```python
from build123d import *

# Parameters (mm, degrees)
SKETCH1_W           = 86.36
SKETCH1_H           = 86.36
BOSS_EXTRUDE1_DEPTH = 43.18
SKETCH2_W           = 81.28
SKETCH2_H           = 81.28
CUT_EXTRUDE2_DEPTH  = 35.56
SKETCH6_W           = 81.28
SKETCH6_H           = 81.28
SKETCH6_R           = 1.016
BOSS_EXTRUDE2_DEPTH = 30.48
SKETCH9_R           = 6.35
CUT_EXTRUDE3_DEPTH  = 5.08
CUT_EXTRUDE4_REACH  = 107.769
SKETCH10_R          = 1.905


with BuildPart() as part:
    # Sketch1 → Boss-Extrude1 (new body)
    with BuildSketch(Plane(origin=(0, 0, 0), x_dir=(1, 0, 0), z_dir=(0, 1, 0))):
        Rectangle(SKETCH1_W, SKETCH1_H)
    extrude(amount=-BOSS_EXTRUDE1_DEPTH)

    # Sketch2 → Cut-Extrude2 (cut)
    with BuildSketch(Plane(origin=(0, -43.18, 0), x_dir=(-1, 0, 0), z_dir=(0, -1, 0))):
        Rectangle(SKETCH2_W, SKETCH2_H)
    extrude(amount=-CUT_EXTRUDE2_DEPTH, mode=Mode.SUBTRACT)

    # Sketch6 → Boss-Extrude2 (add)
    with BuildSketch(Plane(origin=(0, -7.62, 0), x_dir=(-1, 0, 0), z_dir=(0, -1, 0))):
        Rectangle(SKETCH6_W, SKETCH6_H)
        with Locations(Location((-35.56, 35.56, 0), (0, 0, 270))):
            Circle(SKETCH6_R, mode=Mode.SUBTRACT)
        with Locations(Location((35.56, 35.56, 0), (0, 0, 270))):
            Circle(SKETCH6_R, mode=Mode.SUBTRACT)
        with Locations(Location((35.56, -35.56, 0), (0, 0, 270))):
            Circle(SKETCH6_R, mode=Mode.SUBTRACT)
        with Locations(Location((-35.56, -35.56, 0), (0, 0, 270))):
            Circle(SKETCH6_R, mode=Mode.SUBTRACT)
        with BuildLine():
            Line((-27.94, 38.1), (27.94, 38.1))
            ThreePointArc((27.94, 38.1), (29.736051224, 37.356051224), (30.48, 35.56))
            ThreePointArc((30.48, 35.56), (31.967897552, 31.967897552), (35.56, 30.48))
            ThreePointArc((35.56, 30.48), (37.356051224, 29.736051224), (38.1, 27.94))
            Line((38.1, 27.94), (38.1, -27.94))
            ThreePointArc((38.1, -27.94), (37.356051224, -29.736051224), (35.56, -30.48))
            ThreePointArc((35.56, -30.48), (31.967897552, -31.967897552), (30.48, -35.56))
            ThreePointArc((30.48, -35.56), (29.736051224, -37.356051224), (27.94, -38.1))
            Line((27.94, -38.1), (-27.94, -38.1))
            ThreePointArc((-27.94, -38.1), (-29.736051224, -37.356051224), (-30.48, -35.56))
            ThreePointArc((-30.48, -35.56), (-31.967897552, -31.967897552), (-35.56, -30.48))
            ThreePointArc((-35.56, -30.48), (-37.356051224, -29.736051224), (-38.1, -27.94))
            Line((-38.1, -27.94), (-38.1, 27.94))
            ThreePointArc((-38.1, 27.94), (-37.356051224, 29.736051224), (-35.56, 30.48))
            ThreePointArc((-35.56, 30.48), (-31.967897552, 31.967897552), (-30.48, 35.56))
            ThreePointArc((-30.48, 35.56), (-29.736051224, 37.356051224), (-27.94, 38.1))
        make_face(mode=Mode.SUBTRACT)
    extrude(amount=BOSS_EXTRUDE2_DEPTH)

    # Sketch9 → Cut-Extrude3 (cut)
    with BuildSketch(Plane.ZY.offset(43.18)):
        with Locations((0, -27.94)):
            Circle(SKETCH9_R)
        with Locations((-17.78, -18.102622301)):
            Circle(SKETCH9_R)
        with Locations((17.78, -18.102622301)):
            Circle(SKETCH9_R)
    extrude(amount=-CUT_EXTRUDE3_DEPTH, mode=Mode.SUBTRACT)

    # Sketch10 → Cut-Extrude4 (cut, up to next)
    with BuildSketch(Plane.ZY.offset(43.18), mode=Mode.PRIVATE) as cut_extrude4_sk1:
        with Locations((0, -10.16)):
            Circle(SKETCH10_R)
    cut_extrude4_tool1 = extrude(cut_extrude4_sk1.sketch, amount=-CUT_EXTRUDE4_REACH, mode=Mode.PRIVATE) & part.part
    add(cut_extrude4_tool1.solids().sort_by_distance((-43.18, -10.16, 0))[0], mode=Mode.SUBTRACT)


solid = part.part
```
Can you work these out from the model? Positions are in its coordinate system, mm. A direction names the side the tool comes from. Give positions to 0.01 mm unless a question says otherwise; leave off trailing zeros. Order: outer loops, then holes, each group sorted by start corner. A loop starts at its lowest first (then second) coordinate and runs counter-clockwise, first axis right, second up. Notation, with made-up numbers: M 27.25,68.25 L 59.25,68.25 A24 ccw 59.25,81.25 Z; hole C 37.5,56 d1. An arc over 180 degrees is marked long. Write item = value, one per line. Start each with the question number.
Q1. We'd pull the mould along Y, two halves only. Please class faces 1 (the cylindrical face through (-29.756, -22.647, 37.336)), 2 (the flat face through (1, -7.62, -1)), 3 (the cylindrical face through (-40.68, -16.2, 23.84)): pulls with the +Y half, pulls with the -Y half, needs draft (parallel to the pull), parting line crosses it, or undercut.
Q2. Suppose I cut it at A-A (z = -17.78). Write out the boundary of the cut face in (x, y), plus the area to 3 significant figures.
Q3. I need wall thicknesses on probe 1 along Y at (x, z) = (-40, 0) (3 decimals); probe 2 along Z at (x, y) = (35.56, -25.5); probe 3 along Z at (x, y) = (-21.5, -25). Which ranges of each line are inside material? Lowest first, please. Write a range as [from, to].
Q4. For faces 4 (the cylindrical face through (-40.68, -13.81, -22.46)), 5 (the flat face through (1, -41, 40.64)), 6 (the flat face through (-1, -21, -43.18)), which set-ups out of +Z, -Z, +X, -X, +Y, -Y let a thin tool reach every point of the face, with its end or its side?
Q5. Suppose I cut it at B-B (y = -10.16). Write out the boundary of the cut face in (x, z) (3 decimals), plus the area to 3 significant figures.
Q6. Suppose I cut it at C-C (z = 0). Write out the boundary of the cut face in (x, y) (3 decimals).
Q7. Will these pins go through, and if not, where does the flat tip stop? pin 1 Ø2.5 at (x, z) = (-35.56, 35.56) entering from -Y; pin 2 Ø16.5 at (y, z) = (-18.1, -17.78) entering from -X; pin 3 Ø0.6 at (x, z) = (-35.5, 36) entering from -Y; pin 4 Ø10 at (y, z) = (-18.1, 17.78) entering from -X.
Q8. Suppose I cut it at D-D (x = 24). Write out the boundary of the cut face in (y, z).
Check result:
q1.face_1 = needs draft
q1.face_2 = pulls with the -Y half
q1.face_3 = undercut
q2.outline = M -43.18,-43.18 L -40.64,-43.18 L -40.64,-38.1 L -38.1,-38.1 L -38.1,-24.45 L -43.18,-24.45 Z; M -43.18,-11.75 L -38.1,-11.75 L -38.1,-7.62 L 38.1,-7.62 L 38.1,-38.1 L 40.64,-38.1 L 40.64,-43.18 L 43.18,-43.18 L 43.18,0 L -43.18,0 Z
q2.area = 929 mm2
q3.probe_1 = [-38.1, -34.29], [-21.59, -12.065], [-8.255, 0]
q3.probe_2 = [-43.18, -36.58], [-34.54, -30.48], [30.48, 34.54], [36.58, 43.18]
q3.probe_3 = [-43.18, -38.1], [38.1, 43.18]
q4.face_4 = -X
q4.face_5 = -Y
q4.face_6 = -Z, +X, -X, +Y, -Y
q5.outline = M -43.18,-43.18 L 43.18,-43.18 L 43.18,43.18 L -43.18,43.18 L -43.18,1.905 L -38.1,1.905 L -38.1,27.94 A2.54 cw -35.56,30.48 A5.08 ccw -30.48,35.56 A2.54 cw -27.94,38.1 L 27.94,38.1 A2.54 cw 30.48,35.56 A5.08 ccw 35.56,30.48 A2.54 cw 38.1,27.94 L 38.1,-27.94 A2.54 cw 35.56,-30.48 A5.08 ccw 30.48,-35.56 A2.54 cw 27.94,-38.1 L -27.94,-38.1 A2.54 cw -30.48,-35.56 A5.08 ccw -35.56,-30.48 A2.54 cw -38.1,-27.94 L -38.1,-1.905 L -43.18,-1.905 Z; hole C -35.56,-35.56 d2.032; hole C -35.56,35.56 d2.032; hole C 35.56,-35.56 d2.032; hole C 35.56,35.56 d2.032
q5.area = 1,840 mm2
q6.outline = M -43.18,-43.18 L -40.64,-43.18 L -40.64,-38.1 L -38.1,-38.1 L -38.1,-34.29 L -43.18,-34.29 Z; M -43.18,-21.59 L -38.1,-21.59 L -38.1,-12.065 L -43.18,-12.065 Z; M -43.18,-8.255 L -38.1,-8.255 L -38.1,-7.62 L 38.1,-7.62 L 38.1,-38.1 L 40.64,-38.1 L 40.64,-43.18 L 43.18,-43.18 L 43.18,0 L -43.18,0 Z
q7.pin_1 = -38.1
q7.pin_2 = -43.18
q7.pin_3 = -7.62
q7.pin_4 = 38.1
q8.outline = M -43.18,-43.18 L 0,-43.18 L 0,43.18 L -43.18,43.18 L -43.18,40.64 L -38.1,40.64 L -38.1,38.1 L -7.62,38.1 L -7.62,-38.1 L -38.1,-38.1 L -38.1,-40.64 L -43.18,-40.64 Z
